```python
from build123d import *

# Parameters (mm, degrees)
SKETCH1_W           = 182.5
SKETCH1_H           = 35
SKETCH1_R           = 4.125
SKETCH1_R_2         = 1.5
BOSS_EXTRUDE1_DEPTH = 3
CUT_EXTRUDE3_START  = 3.5
SKETCH2_W           = 3
SKETCH2_H           = 9.897866997
SKETCH2_W_2         = 27.5
SKETCH2_W_3         = 2
CUT_EXTRUDE3_DEPTH  = 9


with BuildPart() as part:
    # Sketch1 → Boss-Extrude1 (new body)
    with BuildSketch(Plane(origin=(0, 0, 0), x_dir=(1, 0, 0), z_dir=(0, 1, 0))):
        with Locations((-8.75, 5)):
            Rectangle(SKETCH1_W, SKETCH1_H)
        with Locations((47.5, 5)):
            Circle(SKETCH1_R, mode=Mode.SUBTRACT)
        with Locations((74.5, 5)):
            Circle(SKETCH1_R_2, mode=Mode.SUBTRACT)
        with Locations((20.5, 5)):
            Circle(SKETCH1_R_2, mode=Mode.SUBTRACT)
        with Locations((-97, -9.5)):
            Circle(SKETCH1_R_2, mode=Mode.SUBTRACT)
        with Locations((-97, -3)):
            Circle(SKETCH1_R_2, mode=Mode.SUBTRACT)
        with Locations((-91.5, 8)):
            Circle(SKETCH1_R_2, mode=Mode.SUBTRACT)
        with Locations((-64, 8)):
            Circle(SKETCH1_R_2, mode=Mode.SUBTRACT)
        with Locations((-64, 1)):
            Circle(SKETCH1_R_2, mode=Mode.SUBTRACT)
        with Locations((-91.5, 1)):
            Circle(SKETCH1_R_2, mode=Mode.SUBTRACT)
    extrude(amount=BOSS_EXTRUDE1_DEPTH)

    # Sketch2 → Cut-Extrude3 (cut)
    with BuildSketch(Plane.XY.offset(CUT_EXTRUDE3_START)):
        with Locations((-90.5, 1.550857661)):
            Rectangle(SKETCH2_W, SKETCH2_H)
        with Locations((-75.25, 1.550857661)):
            Rectangle(SKETCH2_W_2, SKETCH2_H)
        with Locations((-93, 1.550857661)):
            Rectangle(SKETCH2_W_3, SKETCH2_H)
    extrude(amount=CUT_EXTRUDE3_DEPTH, mode=Mode.SUBTRACT)


solid = part.part
```
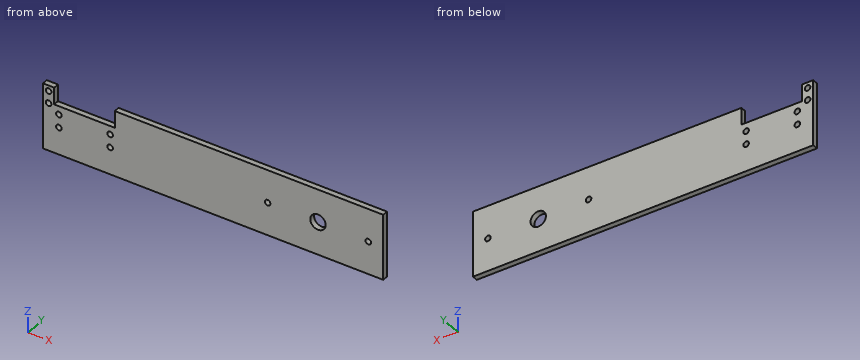
Read the model definition and answer for the solid it produces. Units are mm, in the model's axes. Coordinates: 2 decimals unless noted, no trailing zeros. Write each loop counter-clockwise with the first axis right and the second up, starting at its lowest first coordinate (ties: lowest second). Pieces come first, ordered by that corner, then holes. Notation, with made-up numbers: (13, -31) -> (49, -31) arc R23 ccw to (49, -18) -> close; hole circle Ø10 at (51, -33). An arc over 180 degrees is marked (long way). Answer as a JSON object with one key per item and string values.
Q1. The part is cut by section D-D on x = 74.5. Give the vertices of the cut face in (y, z), then the cut area to 3 significant figures.
The answers:
{"outline": "(0, -22.5) -> (3, -22.5) -> (3, -6.5) -> (0, -6.5) -> close; (0, -3.5) -> (3, -3.5) -> (3, 12.5) -> (0, 12.5) -> close", "area": "96.0 mm2"}
Q2. Consider line 1 (X direction, y = 2.85, z = -5) (3 decimals); line 2 (Z direction, x = -64, y = 2.2); line 3 (Z direction, x = -97, y = 1.75). Determine where each line is inside the solid, lowest interval first. Write a range as [from, to].
The answers:
{"line 1": "x = [-100, 19], [22, 43.375], [51.625, 73], [76, 82.5]", "line 2": "z = [-22.5, -9.5], [-6.5, -2.5], [0.5, 3.5]", "line 3": "z = [-22.5, 1.5], [4.5, 8], [11, 12.5]"}
Q3. The part is cut by section A-A on z = 9.5. Give the vertices of the cut face in (x, y).
The answers:
{"outline": "(-100, 0) -> (-98.5, 0) -> (-98.5, 3) -> (-100, 3) -> close; (-95.5, 0) -> (-94, 0) -> (-94, 3) -> (-95.5, 3) -> close; (-61.5, 0) -> (82.5, 0) -> (82.5, 3) -> (-61.5, 3) -> close"}
Q4. The part is cut by section C-C on y = 0.6. Give the number of separate pieces and of enclosed holes in the cut face, then the cut area to 4 significant figures.
The answers:
{"separate pieces": "1", "enclosed holes": "9", "area": "5,985 mm2"}
Q5. The part is cut by section B-B on x = -97. Give the vertices of the cut face in (y, z).
The answers:
{"outline": "(0, -22.5) -> (3, -22.5) -> (3, 1.5) -> (0, 1.5) -> close; (0, 4.5) -> (3, 4.5) -> (3, 8) -> (0, 8) -> close; (0, 11) -> (3, 11) -> (3, 12.5) -> (0, 12.5) -> close"}
Q6. Flat-ended cylindrical pins translate along their axes: pin 1 Ø5 at (x, z) = (-91.5, -1) entering from -Y; pin 2 Ø2.5 at (x, z) = (74.5, -5) entering from -Y (1 decimal); pin 3 Ø0.9 at (x, y) = (-76.5, 1) entering from +Z. Find the tip coordinate at first contact, or state that the pin passes through.
The answers:
{"pin 1": "stops at y = 0", "pin 2": "passes through", "pin 3": "stops at z = 3.5"}
